Drawing for the job (mm, zero at the part's lowest x, y, z). Round coordinates to 2 decimals unless told otherwise and drop trailing zeros. Write each loop counter-clockwise with the first axis right and the second up, starting at its lowest first coordinate (ties: lowest second). Pieces come first, ordered by that corner, then holes. Notation, with made-up numbers: M -5,50.5 L 15,50.5 A19 cw 15,79.5 Z; hole C -25,18 d8. An arc over 180 degrees is marked long. Use a Markdown table: item, result.
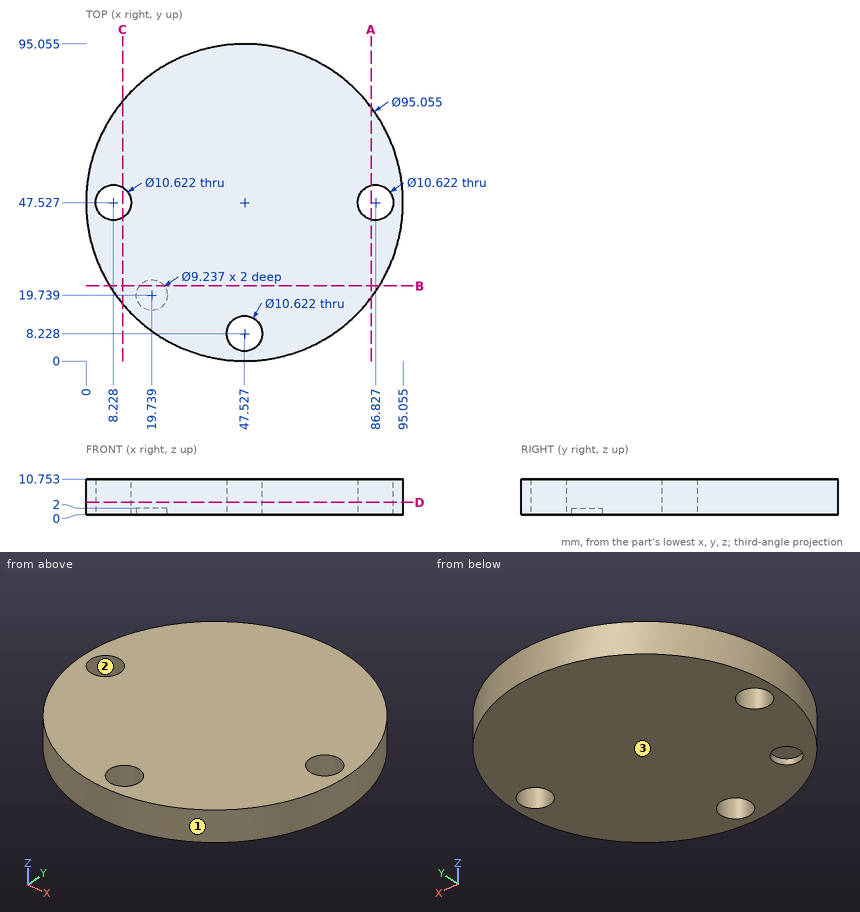
Q1. Cut at B-B on y = 22.5. Give the cut face in (x, z), and give its area (3 significant figures).
Response values:
| item | result |
|---|---|
| outline | M 7.12,0 L 16.04,0 L 16.04,2 L 23.44,2 L 23.44,0 L 87.93,0 L 87.93,10.75 L 7.12,10.75 Z |
| area | 854 mm2 |
Q2. Cut at C-C on x = 11. Give the cut face in (y, z) (1 decimal).
Response values:
| item | result |
|---|---|
| outline | M 17.1,0 L 43,0 L 43,10.8 L 17.1,10.8 Z; M 52.1,0 L 77.9,0 L 77.9,10.8 L 52.1,10.8 Z |
Q3. Cut at A-A on x = 85.5. Give the cut face in (y, z) (1 decimal).
Response values:
| item | result |
|---|---|
| outline | M 18.9,0 L 42.4,0 L 42.4,10.8 L 18.9,10.8 Z; M 52.7,0 L 76.1,0 L 76.1,10.8 L 52.7,10.8 Z |
Q4. Drill centre lines: L1, parallel to X at y = 49, z = 6.75 (1 decimal); L2, parallel to Y at x = 46, z = 3 (1 decimal); L3, parallel to Y at x = 4, z = 3 (1 decimal). Where is each one in solid material? Low to high.
Response values:
| item | result |
|---|---|
| L1 | x = 0 to 3.1, 13.3 to 81.7, 91.9 to 95 |
| L2 | y = 0 to 3.1, 13.3 to 95 |
| L3 | y = 28.4 to 44.3, 50.7 to 66.6 |
Q5. Cut at D-D on z = 3.75. Give the cut face in (x, y) (1 decimal), and give its area (3 significant figures).
Response values:
| item | result |
|---|---|
| outline | C 47.5,47.5 d95.1; hole C 8.2,47.5 d10.6; hole C 47.5,8.2 d10.6; hole C 86.8,47.5 d10.6 |
| area | 6,830 mm2 |
Q6. Drop flat-ended pins along their axis: P1, Ø4, axis at y = 19.5, z = 6.5, coming from the -X side; P2, Ø5, axis at x = 81, z = 1.5, coming from the +Y side (1 decimal); P3, Ø5, axis at x = 37, z = 2.5, coming from the +Y side. Give the stop position or say it passes through.
Response values:
| item | result |
|---|---|
| P1 | stops at x = 7.76 |
| P2 | stops at y = 83.6 |
| P3 | stops at y = 94.37 |
Q7. Two-plate mould, pull along Y, no slides. Class the marked faces 1, 2 and 3: +Y half, -Y half, draft (parallel to the pull), parting line (faces both ways), or undercut.
Response values:
| item | result |
|---|---|
| face 1 | parting line |
| face 2 | undercut |
| face 3 | draft |
